The figure shows three views and two pictorial views of one solid part (mm, origin at its lowest corner). Answer the questions. Coordinates: 2 decimals unless noted, no trailing zeros. Write each loop counter-clockwise with the first axis right and the second up, starting at its lowest first coordinate (ties: lowest second). Pieces come first, ordered by that corner, then holes.
Item 1: Section A-A (z = 6.5) is taken. Give the vertices of the cut face in (x, y).
Item 2: Section C-C (y = 1.7) is taken. Give the vertices of the cut face in (x, z), then the cut area to 3 significant figures.
Item 3: Straight lines are drawn through the part: probe 1 along X at (y, z) = (0.95, 6.5); probe 2 along Z at (x, y) = (10, 2); probe 3 along X at (y, z) = (2.4, 9). For each, find the intervals that lie inside material, in ascending order.
Item 4: Section B-B (x = 10) is taken. Give the vertices of the cut face in (y, z).
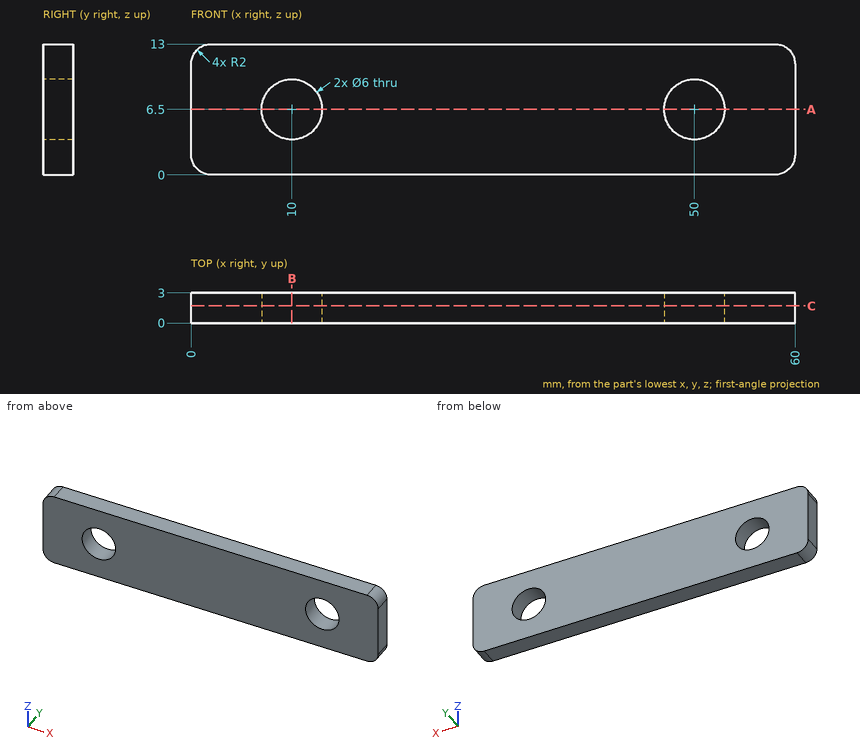
Established:
1. outline: (0, 0) - (7, 0) - (7, 3) - (0, 3) - close; (13, 0) - (47, 0) - (47, 3) - (13, 3) - close; (53, 0) - (60, 0) - (60, 3) - (53, 3) - close
2. outline: (0, 2) arc R2 ccw to (2, 0) - (58, 0) arc R2 ccw to (60, 2) - (60, 11) arc R2 ccw to (58, 13) - (2, 13) arc R2 ccw to (0, 11) - close; hole circle Ø6 at (10, 6.5); hole circle Ø6 at (50, 6.5)
2. area: 720 mm2
3. probe 1: x = 0 to 7, 13 to 47, 53 to 60
3. probe 2: z = 0 to 3.5, 9.5 to 13
3. probe 3: x = 0 to 8.34, 11.66 to 48.34, 51.66 to 60
4. outline: (0, 0) - (3, 0) - (3, 3.5) - (0, 3.5) - close; (0, 9.5) - (3, 9.5) - (3, 13) - (0, 13) - close
